from build123d import *

# Parameters (mm, degrees)
SKETCH_1_W      = 55
SKETCH_1_H      = 20
SKETCH_1_R      = 2.1
SKETCH_1_R_2    = 20
SKETCH_1_R_3    = 11
EXTRUDE_1_DEPTH = 3
FILLET_1_R      = 2


with BuildPart() as part:
    # ｽｹｯﾁ1 → ﾎﾞｽ - 押し出し1 (new body)
    # profile 1 of 4: a face of its own
    with BuildSketch(Plane.XY):
        Rectangle(SKETCH_1_W, SKETCH_1_H)
        with Locations((22.5, 0)):
            Circle(SKETCH_1_R, mode=Mode.SUBTRACT)
        with Locations((-22.5, 0)):
            Circle(SKETCH_1_R, mode=Mode.SUBTRACT)
    # profile 2 of 4: a face of its own
    with BuildSketch(Plane.XY):
        with BuildLine():
            Line((1.9e-08, -10), (-27.5, -10))
            Line((-27.5, -10), (-19.027027027, -36.162162162))
            ThreePointArc((-19.027027027, -36.162162162), (-16.174721681, -18.236566039), (1.9e-08, -10))
        make_face()
    # profile 3 of 4: a face of its own
    with BuildSketch(Plane.XY):
        with Locations((0, -30)):
            Circle(SKETCH_1_R_2)
        with Locations((0, -30)):
            Circle(SKETCH_1_R_3, mode=Mode.SUBTRACT)
    # profile 4 of 4: a face of its own
    with BuildSketch(Plane.XY):
        with BuildLine():
            Line((19.027027027, -36.162162162), (27.5, -10))
            Line((27.5, -10), (1.9e-08, -10))
            ThreePointArc((1.9e-08, -10), (14.14213563, -15.857864383), (20, -30))
            ThreePointArc((20, -30), (19.755259307, -33.119251469), (19.027027027, -36.162162162))
        make_face()
    extrude(amount=EXTRUDE_1_DEPTH)

    # ﾌｨﾚｯﾄ1
    fillet_1_edges = [part.edges().sort_by_distance(p)[0] for p in [
        (27.5, -10, 1.5),
        (-27.5, -10, 1.5),
        (-27.5, 10, 1.5),
        (27.5, 10, 1.5),
    ]]
    fillet(fillet_1_edges, radius=FILLET_1_R)


solid = part.part
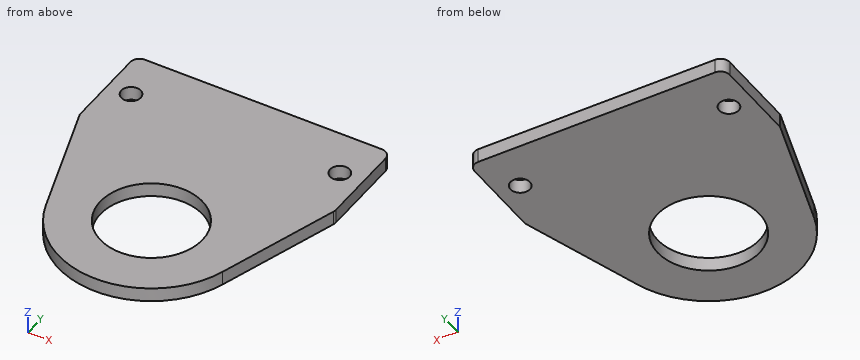
Part model, mm, in its own coordinate system. Give positions to 0.01 mm unless a question says otherwise; leave off trailing zeros. Loops run counter-clockwise (first coordinate to the right, second up) from the corner with the lowest first, then second, coordinate; pieces in that order, holes last. Notation, with made-up numbers: (45.5, -7.5) -> (78.5, -7.5) arc R25 ccw to (78.5, 18.5) -> close; hole circle Ø10 at (87.5, -20). An arc over 180 degrees is marked (long way). Write each question's results on one line, items separated by ' | '. Start each with the question number.
Q1. Band-saw the part on A-A on y = 0. List the corners of the cut face in (x, z).
Q2. Band-saw the part on C-C on z = 2.5. List the corners of the cut face in (x, y).
Q3. Pin check, flat tips, straight feed: P1, Ø8, axis at x = -21, y = -25, coming from the -Z side; P2, Ø1, axis at x = -10, z = 0.5, coming from the -Y side. Stop position of each tip, or through.
Q4. Band-saw the part on D-D on y = -37. List the corners of the cut face in (x, z) (3 decimals).
Q5. Wall check: L1, parallel to X at y = -31.5, z = 2.55; L2, parallel to Y at x = 10, z = 2.2; L3, parallel to X at y = -43, z = 0.6. Give the ranges that are in metal, low to high.
Q6. Band-saw the part on B-B on x = 0. List the corners of the cut face in (y, z), plus the area to 3 significant figures.
Results are:
1) outline: (-27.5, 0) -> (-24.6, 0) -> (-24.6, 3) -> (-27.5, 3) -> close; (-20.4, 0) -> (20.4, 0) -> (20.4, 3) -> (-20.4, 3) -> close; (24.6, 0) -> (27.5, 0) -> (27.5, 3) -> (24.6, 3) -> close
2) outline: (-27.5, -9.68) arc R2 ccw to (-27.4, -10.3) -> (-19.03, -36.16) arc R20 ccw to (19.03, -36.16) -> (27.4, -10.3) arc R2 ccw to (27.5, -9.68) -> (27.5, 8) arc R2 ccw to (25.5, 10) -> (-25.5, 10) arc R2 ccw to (-27.5, 8) -> close; hole circle Ø4.2 at (-22.5, 0); hole circle Ø22 at (0, -30); hole circle Ø4.2 at (22.5, 0)
3) P1: stops at z = 0 | P2: stops at y = -47.6
4) outline: (-18.735, 0) -> (-8.485, 0) -> (-8.485, 3) -> (-18.735, 3) -> close; (8.485, 0) -> (18.735, 0) -> (18.735, 3) -> (8.485, 3) -> close
5) L1: x = -20.54 to -10.9, 10.9 to 20.54 | L2: y = -47.32 to -34.58, -25.42 to 10 | L3: x = -15.2 to 15.2
6) outline: (-50, 0) -> (-41, 0) -> (-41, 3) -> (-50, 3) -> close; (-19, 0) -> (10, 0) -> (10, 3) -> (-19, 3) -> close | area: 114 mm²
